```python
from build123d import *

# Parameters (mm, degrees)
SKETCH1_R               = 2.8
BOSS_EXTRUDE1_DEPTH     = 5
CUT_EXTRUDE1_DEPTH      = 16
CUT_EXTRUDE1_DEPTH_BACK = 10
SKETCH2_R               = 1.75
CUT_EXTRUDE2_DEPTH      = 3.5
BOSS_EXTRUDE2_DEPTH     = 6
SKETCH5_R               = 1.75
CUT_EXTRUDE3_DEPTH      = 58.313311378


with BuildPart() as part:
    # Sketch1 → Boss-Extrude1 (new body)
    with BuildSketch(Plane(origin=(0, 0, 0), x_dir=(1, 0, 0), z_dir=(0, 1, 0))):
        Polygon((-40.303943114, 15.555205773), (-15.555205773, 40.303943114), (4.694794227, 40.303943114), (24.042773974, 20.955963368), (24.042773974, 0.705963368), (-0.705963368, -24.042773974), (-20.955963368, -24.042773974), (-40.303943114, -4.694794227), align=None)
        with Locations(Location((-11.666118476, -16.618152771, 0), (0, 0, 270))):
            Circle(SKETCH1_R, mode=Mode.SUBTRACT)
        with Locations(Location((16.618152771, 11.666118476, 0), (0, 0, 270))):
            Circle(SKETCH1_R, mode=Mode.SUBTRACT)
        with Locations(Location((-4.595050664, 32.879321912, 0), (0, 0, 270))):
            Circle(SKETCH1_R, mode=Mode.SUBTRACT)
        with Locations(Location((-32.879321912, 4.595050664, 0), (0, 0, 270))):
            Circle(SKETCH1_R, mode=Mode.SUBTRACT)
    extrude(amount=BOSS_EXTRUDE1_DEPTH)

    # Sketch2 → Cut-Extrude1 (cut, two sides: drawn at the far end of the back side and taken through both)
    with BuildSketch(Plane(origin=(0, 5, 0), x_dir=(1, 0, 0), z_dir=(0, 1, 0)).offset(-CUT_EXTRUDE1_DEPTH_BACK)):
        with Locations(Location((13.966502342, 3.711167188, 0), (0, 0, 90))):
            Circle(SKETCH2_R)
        with Locations(Location((-3.711167188, -13.966502342, 0), (0, 0, 90))):
            Circle(SKETCH2_R)
        with Locations(Location((-21.31812604, 21.31812604, 0), (0, 0, 90))):
            Circle(SKETCH2_R)
    extrude(amount=CUT_EXTRUDE1_DEPTH + CUT_EXTRUDE1_DEPTH_BACK, mode=Mode.SUBTRACT)

    # Sketch3 → Cut-Extrude2 (cut)
    with BuildSketch(Plane.XZ):
        Polygon((-4.562913887, 10.787740387), (-1.384151932, 11.639487086), (-0.532405234, 14.81824904), (-2.859420489, 17.145264296), (-6.038182444, 16.293517597), (-6.889929142, 13.114755643), align=None)
        Polygon((10.787740387, -4.562913887), (13.114755643, -6.889929142), (16.293517597, -6.038182444), (17.145264296, -2.859420489), (14.81824904, -0.532405234), (11.639487086, -1.384151932), align=None)
        Polygon((-22.169872738, -24.496887994), (-18.991110784, -23.645141295), (-18.139364085, -20.466379341), (-20.466379341, -18.139364085), (-23.645141295, -18.991110784), (-24.496887994, -22.169872738), align=None)
    extrude(amount=-CUT_EXTRUDE2_DEPTH, mode=Mode.SUBTRACT)

    # Sketch4 → Boss-Extrude2 (add)
    with BuildSketch(Plane(origin=(0, 5, 0), x_dir=(1, 0, 0), z_dir=(0, 1, 0))):
        Polygon((-7.246701094, -13.966502342), (-3.711167188, -17.502036248), (-0.175633282, -13.966502342), (-3.711167188, -10.430968436), align=None)
        Polygon((-21.31812604, 17.782592134), (-24.853659945, 21.31812604), (-21.31812604, 24.853659945), (-17.782592134, 21.31812604), align=None)
        Polygon((10.430968436, 3.711167188), (13.966502342, 7.246701094), (17.502036248, 3.711167188), (13.966502342, 0.175633282), align=None)
    extrude(amount=BOSS_EXTRUDE2_DEPTH)

    # Sketch5 → Cut-Extrude3 (cut, through all)
    with BuildSketch(Plane.XZ.offset(-5)):
        with Locations(Location((-21.31812604, -21.31812604, 0), (0, 0, 270))):
            Circle(SKETCH5_R)
        with Locations(Location((-3.711167188, 13.966502342, 0), (0, 0, 270))):
            Circle(SKETCH5_R)
        with Locations(Location((13.966502342, -3.711167188, 0), (0, 0, 270))):
            Circle(SKETCH5_R)
    extrude(amount=-CUT_EXTRUDE3_DEPTH, mode=Mode.SUBTRACT)


solid = part.part
```
Here's how the part is built. I have some questions about the finished solid (model axes, mm). A direction names the side the tool comes from. Coordinates: 2 decimals unless noted, no trailing zeros. Order: outer loops, then holes, each group sorted by start corner. A loop starts at its lowest first (then second) coordinate and runs counter-clockwise, first axis right, second up.
1) Imagine slicing it at B-B on x = -34. List the corners of the cut face in (y, z) for me.
2) We'd pull the mould along Z, two halves only. Please class faces 5 (the face through (-23.11, 7.96, -23.06)), 6 (the face through (-5.667, 2.465, -30.293)), 7 (the face through (11.842, 2.465, 11.495)): +Z half, -Z half, draft (parallel to the pull), parting line (faces both ways), or undercut.
3) Will these pins go through, and if not, where does the flat tip stop? pin 1 (4.5 mm diameter, centred on x = -21.32, z = -21.32, fed in from -Y); pin 2 (4 mm diameter, centred on x = -21, y = 5.5, fed in from -Z); pin 3 (9 mm diameter, centred on x = 16.62, z = -11.67, fed in from +Y); pin 4 (3.5 mm diameter, centred on x = -4.6, z = -32.88, fed in from -Y).
4) I need wall thicknesses on line 1 (Y direction, x = -33, z = 5); line 2 (Z direction, x = 13, y = 7.75); line 3 (Z direction, x = -23.5, y = 0.75). Which ranges of each line are inside material? Lowest first, please.
5) Imagine slicing it at C-C on z = -34. List the corners of the cut face in (x, y) for me.
6) Imagine slicing it at A-A on y = 7.5. List the corners of the cut face in (x, z) for me, and give its area (3 significant figures).
7) Which directions (+Z, -Z, +X, -X, +Y, -Y) give clear straight access to the entire face, cutting with the end or side of a thin tool? Please do faces 1 (the face through (12.17, 7.96, -5.45)), 2 (the face through (-8, 5, -9)), 3 (the face through (-19.5, 8, -19.6)), 4 (the face through (13.251, 1.726, -0.952)).
8) Imagine slicing it at D-D on y = 1. State how many separate pieces and enclosed holes the cut face has, and give its area (3 significant figures).
Response values:
1. outline: (0, -21.86) - (5, -21.86) - (5, -7.16) - (0, -7.16) - close; (0, -2.03) - (5, -2.03) - (5, 11) - (0, 11) - close
2. face 5: -Z half
2. face 6: undercut
2. face 7: +Z half
3. pin 1: stops at y = 3.5
3. pin 2: stops at z = -36.8
3. pin 3: stops at y = 5
3. pin 4: passes through
4. line 1: y = 0 to 5
4. line 2: z = -6.28 to -5.17, -2.25 to -1.14
4. line 3: z = -32.36 to -23.17, -18.95 to 21.5
5. outline: (-21.86, 0) - (-7.16, 0) - (-7.16, 5) - (-21.86, 5) - close; (-2.03, 0) - (11, 0) - (11, 5) - (-2.03, 5) - close
6. outline: (-24.85, -21.32) - (-21.32, -24.85) - (-17.78, -21.32) - (-21.32, -17.78) - close; (-7.25, 13.97) - (-3.71, 10.43) - (-0.18, 13.97) - (-3.71, 17.5) - close; (10.43, -3.71) - (13.97, -7.25) - (17.5, -3.71) - (13.97, -0.18) - close; hole circle Ø3.5 at (-21.32, -21.32); hole circle Ø3.5 at (-3.71, 13.97); hole circle Ø3.5 at (13.97, -3.71)
6. area: 46.1 mm2
7. face 1: -Z, -X, +Y
7. face 2: +Y
7. face 3: +Z, +X, +Y
7. face 4: -Y
8. separate pieces: 1
8. enclosed holes: 7
8. area: 2,970 mm2
